from build123d import *

# Parameters (mm, degrees)
F0_R     = 6.35
F1_DEPTH = 3.81


with BuildPart() as f1:
    # F0 (on Top) → F1 (new body, symmetric)
    with BuildSketch(Plane.XY):
        with BuildLine():
            Line((-25.978442, -31.237892), (-24.182391, -29.441841))
            ThreePointArc((-24.182391, -29.441841), (-21.167226, -31.678992), (-17.946514, -33.60852))
            Line((-17.946514, -33.60852), (-18.91853, -35.955174))
            Line((-18.91853, -35.955174), (-19.883203, -40.701224))
            Line((-19.883203, -40.701224), (-17.301883, -41.770441))
            Line((-17.301883, -41.770441), (-14.720564, -42.839659))
            Line((-14.720564, -42.839659), (-12.046727, -38.801568))
            Line((-12.046727, -38.801568), (-11.074711, -36.454914))
            ThreePointArc((-11.074711, -36.454914), (-7.432941, -37.367919), (-3.718993, -37.918058))
            Line((-3.718993, -37.918058), (-3.718993, -40.458058))
            Line((-3.718993, -40.458058), (-2.794, -45.212))
            Line((-2.794, -45.212), (0, -45.212))
            Line((0, -45.212), (2.794, -45.212))
            Line((2.794, -45.212), (3.718993, -40.458058))
            Line((3.718993, -40.458058), (3.718993, -37.918058))
            ThreePointArc((3.718993, -37.918058), (7.432941, -37.367919), (11.074711, -36.454914))
            Line((11.074711, -36.454914), (12.046727, -38.801568))
            Line((12.046727, -38.801568), (14.720564, -42.839659))
            Line((14.720564, -42.839659), (17.301883, -41.770441))
            Line((17.301883, -41.770441), (19.883203, -40.701224))
            Line((19.883203, -40.701224), (18.91853, -35.955174))
            Line((18.91853, -35.955174), (17.946514, -33.60852))
            ThreePointArc((17.946514, -33.60852), (21.167226, -31.678992), (24.182391, -29.441841))
            Line((24.182391, -29.441841), (25.978442, -31.237892))
            Line((25.978442, -31.237892), (29.994055, -33.945368))
            Line((29.994055, -33.945368), (31.969712, -31.969712))
            Line((31.969712, -31.969712), (33.945368, -29.994055))
            Line((33.945368, -29.994055), (31.237892, -25.978442))
            Line((31.237892, -25.978442), (29.441841, -24.182391))
            ThreePointArc((29.441841, -24.182391), (31.678992, -21.167226), (33.60852, -17.946514))
            Line((33.60852, -17.946514), (35.955174, -18.91853))
            Line((35.955174, -18.91853), (40.701224, -19.883203))
            Line((40.701224, -19.883203), (41.770441, -17.301883))
            Line((41.770441, -17.301883), (42.839659, -14.720564))
            Line((42.839659, -14.720564), (38.801568, -12.046727))
            Line((38.801568, -12.046727), (36.454914, -11.074711))
            ThreePointArc((36.454914, -11.074711), (37.367919, -7.432941), (37.918058, -3.718993))
            Line((37.918058, -3.718993), (40.458058, -3.718993))
            Line((40.458058, -3.718993), (45.212, -2.794))
            Line((45.212, -2.794), (45.212, 0))
            Line((45.212, 0), (45.212, 2.794))
            Line((45.212, 2.794), (40.458058, 3.718993))
            Line((40.458058, 3.718993), (37.918058, 3.718993))
            ThreePointArc((37.918058, 3.718993), (37.367919, 7.432941), (36.454914, 11.074711))
            Line((36.454914, 11.074711), (38.801568, 12.046727))
            Line((38.801568, 12.046727), (42.839659, 14.720564))
            Line((42.839659, 14.720564), (41.770441, 17.301883))
            Line((41.770441, 17.301883), (40.701224, 19.883203))
            Line((40.701224, 19.883203), (35.955174, 18.91853))
            Line((35.955174, 18.91853), (33.60852, 17.946514))
            ThreePointArc((33.60852, 17.946514), (31.678992, 21.167226), (29.441841, 24.182391))
            Line((29.441841, 24.182391), (31.237892, 25.978442))
            Line((31.237892, 25.978442), (33.945368, 29.994055))
            Line((33.945368, 29.994055), (31.969712, 31.969712))
            Line((31.969712, 31.969712), (29.994055, 33.945368))
            Line((29.994055, 33.945368), (25.978442, 31.237892))
            Line((25.978442, 31.237892), (24.182391, 29.441841))
            ThreePointArc((24.182391, 29.441841), (21.167226, 31.678992), (17.946514, 33.60852))
            Line((17.946514, 33.60852), (18.91853, 35.955174))
            Line((18.91853, 35.955174), (19.883203, 40.701224))
            Line((19.883203, 40.701224), (17.301883, 41.770441))
            Line((17.301883, 41.770441), (14.720564, 42.839659))
            Line((14.720564, 42.839659), (12.046727, 38.801568))
            Line((12.046727, 38.801568), (11.074711, 36.454914))
            ThreePointArc((11.074711, 36.454914), (7.432941, 37.367919), (3.718993, 37.918058))
            Line((3.718993, 37.918058), (3.718993, 40.458058))
            Line((3.718993, 40.458058), (2.794, 45.212))
            Line((2.794, 45.212), (0, 45.212))
            Line((0, 45.212), (-2.794, 45.212))
            Line((-2.794, 45.212), (-3.718993, 40.458058))
            Line((-3.718993, 40.458058), (-3.718993, 37.918058))
            ThreePointArc((-3.718993, 37.918058), (-7.432941, 37.367919), (-11.074711, 36.454914))
            Line((-11.074711, 36.454914), (-12.046727, 38.801568))
            Line((-12.046727, 38.801568), (-14.720564, 42.839659))
            Line((-14.720564, 42.839659), (-17.301883, 41.770441))
            Line((-17.301883, 41.770441), (-19.883203, 40.701224))
            Line((-19.883203, 40.701224), (-18.91853, 35.955174))
            Line((-18.91853, 35.955174), (-17.946514, 33.60852))
            ThreePointArc((-17.946514, 33.60852), (-21.167226, 31.678992), (-24.182391, 29.441841))
            Line((-24.182391, 29.441841), (-25.978442, 31.237892))
            Line((-25.978442, 31.237892), (-29.994055, 33.945368))
            Line((-29.994055, 33.945368), (-31.969712, 31.969712))
            Line((-31.969712, 31.969712), (-33.945368, 29.994055))
            Line((-33.945368, 29.994055), (-31.237892, 25.978442))
            Line((-31.237892, 25.978442), (-29.441841, 24.182391))
            ThreePointArc((-29.441841, 24.182391), (-31.678992, 21.167226), (-33.60852, 17.946514))
            Line((-33.60852, 17.946514), (-35.955174, 18.91853))
            Line((-35.955174, 18.91853), (-40.701224, 19.883203))
            Line((-40.701224, 19.883203), (-41.770441, 17.301883))
            Line((-41.770441, 17.301883), (-42.839659, 14.720564))
            Line((-42.839659, 14.720564), (-38.801568, 12.046727))
            Line((-38.801568, 12.046727), (-36.454914, 11.074711))
            ThreePointArc((-36.454914, 11.074711), (-37.367919, 7.432941), (-37.918058, 3.718993))
            Line((-37.918058, 3.718993), (-40.458058, 3.718993))
            Line((-40.458058, 3.718993), (-45.212, 2.794))
            Line((-45.212, 2.794), (-45.212, 0))
            Line((-45.212, 0), (-45.212, -2.794))
            Line((-45.212, -2.794), (-40.458058, -3.718993))
            Line((-40.458058, -3.718993), (-37.918058, -3.718993))
            ThreePointArc((-37.918058, -3.718993), (-37.367919, -7.432941), (-36.454914, -11.074711))
            Line((-36.454914, -11.074711), (-38.801568, -12.046727))
            Line((-38.801568, -12.046727), (-42.839659, -14.720564))
            Line((-42.839659, -14.720564), (-41.770441, -17.301883))
            Line((-41.770441, -17.301883), (-40.701224, -19.883203))
            Line((-40.701224, -19.883203), (-35.955174, -18.91853))
            Line((-35.955174, -18.91853), (-33.60852, -17.946514))
            ThreePointArc((-33.60852, -17.946514), (-31.678992, -21.167226), (-29.441841, -24.182391))
            Line((-29.441841, -24.182391), (-31.237892, -25.978442))
            Line((-31.237892, -25.978442), (-33.945368, -29.994055))
            Line((-33.945368, -29.994055), (-31.969712, -31.969712))
            Line((-31.969712, -31.969712), (-29.994055, -33.945368))
            Line((-29.994055, -33.945368), (-25.978442, -31.237892))
        make_face()
        Circle(F0_R, mode=Mode.SUBTRACT)
    extrude(amount=F1_DEPTH, both=True)


solid = f1.part
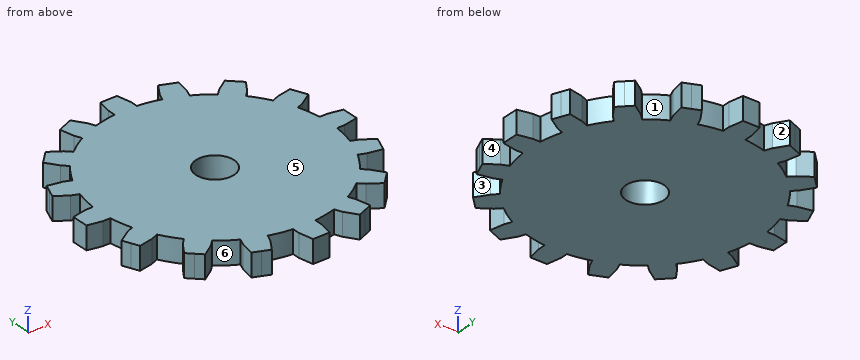
Design review of the part built by this model. Coordinates are the model's own, in mm. Face numbers are marked on the shaded views. A direction names the side the tool comes from. Give positions to 0.01 mm unless a question says otherwise; leave off trailing zeros. Loops run counter-clockwise (first coordinate to the right, second up) from the corner with the lowest first, then second, coordinate; pieces in that order, holes last. Notation, with made-up numbers: (13, 37.5) - (55, 37.5) arc R37 cw to (55, 75.5) - close; hole circle Ø8 at (80, 54.25). An arc over 180 degrees is marked (long way). Write item = value, one per line.
1) Clearance check with flat-ended pins moving along their axes: pin 1 Ø1 at (y, z) = (-15, -2) entering from -X; pin 2 Ø0.8 at (y, z) = (39.5, -1.5) entering from +X; pin 3 Ø1.3 at (x, z) = (39, -1.5) entering from -Y; pin 4 Ø10 at (x, y) = (0, 0) entering from +Z. State where each tip first meets the part, or that it passes through.
Result sheet:
pin_1 = -42.84
pin_2 = 19.72
pin_3 = -19.67
pin_4 = through
2) Tool access review of the marked faces 1, 2 and 3: name each direction out of +Z, -Z, +X, -X, +Y, -Y from which nothing blocks a thin tool from reaching the whole face with its end or side.
Result sheet:
face_1 = +Z, -Z
face_2 = +Z, -Z, +Y
face_3 = +Z, -Z, +X
3) To check wall thickness, follow line 1 (Y direction, x = 0, z = -1); line 2 (Y direction, x = 32, z = 1); line 3 (Y direction, x = 39, z = 3). State the ranges of each line that lie inside material, in increasing order.
Result sheet:
line_1 = -45.21 to -6.35, 6.35 to 45.21
line_2 = -31.94 to -27.11, -20.68 to 20.68, 27.11 to 31.94
line_3 = -19.54 to -12.18, -3.72 to 3.72, 12.18 to 19.54
4) Take a section at A-A on y = 0. State the section outline as (x, z) points.
Result sheet:
outline = (-45.21, -3.81) - (-6.35, -3.81) - (-6.35, 3.81) - (-45.21, 3.81) - close; (6.35, -3.81) - (45.21, -3.81) - (45.21, 3.81) - (6.35, 3.81) - close
5) Draft analysis for pull direction X (two halves, no side actions). For the marked faces 4, 5 and 6, state which applies: +X half, -X half, draft (parallel to the pull), parting line (faces both ways), or undercut.
Result sheet:
face_4 = +X half
face_5 = draft
face_6 = undercut
